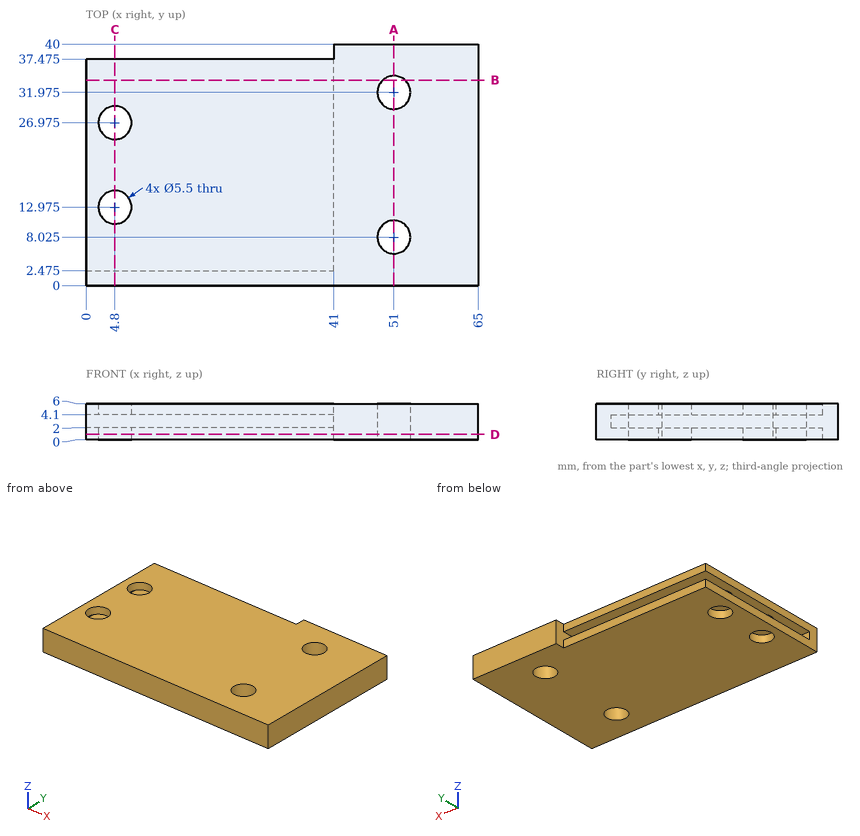
Source: three-view drawing plus pictorial views. Frame: mm from the lowest corner of the part. Give positions to 0.01 mm unless a question says otherwise; leave off trailing zeros. Write each loop counter-clockwise with the first axis right and the second up, starting at its lowest first coordinate (ties: lowest second). Pieces come first, ordered by that corner, then holes. Notation, with made-up numbers: M -4.75,82.25 L 44.25,82.25 A25 ccw 44.25,95.25 Z; hole C 32,49 d10. An arc over 180 degrees is marked long. Use one line per item in the form item = value.
1. Cut plane D-D on z = 0.9. Return loops of the section in (x, y) (3 decimals).
Outcome:
outline = M 0,0 L 65,0 L 65,40 L 41,40 L 41,37.475 L 0,37.475 Z; hole C 4.8,12.975 d5.5; hole C 4.8,26.975 d5.5; hole C 51,8.025 d5.5; hole C 51,31.975 d5.5
2. Cut plane A-A on x = 51. Return loops of the section in (y, z) (3 decimals), and give its area (3 significant figures).
Outcome:
outline = M 0,0 L 5.275,0 L 5.275,6 L 0,6 Z; M 10.775,0 L 29.225,0 L 29.225,6 L 10.775,6 Z; M 34.725,0 L 40,0 L 40,6 L 34.725,6 Z
area = 174 mm²
3. Cut plane C-C on x = 4.8. Return loops of the section in (y, z) (3 decimals), and give its area (3 significant figures).
Outcome:
outline = M 0,0 L 10.225,0 L 10.225,2 L 2.475,2 L 2.475,4.1 L 10.225,4.1 L 10.225,6 L 0,6 Z; M 15.725,0 L 24.225,0 L 24.225,2 L 15.725,2 Z; M 15.725,4.1 L 24.225,4.1 L 24.225,6 L 15.725,6 Z; M 29.725,0 L 37.475,0 L 37.475,2 L 29.725,2 Z; M 29.725,4.1 L 37.475,4.1 L 37.475,6 L 29.725,6 Z
area = 108 mm²
4. Cut plane B-B on y = 34. Return loops of the section in (x, z), and give its area (3 significant figures).
Outcome:
outline = M 0,0 L 49.14,0 L 49.14,6 L 0,6 L 0,4.1 L 41,4.1 L 41,2 L 0,2 Z; M 52.86,0 L 65,0 L 65,6 L 52.86,6 Z
area = 282 mm²
5. First-contact query: P1, Ø5, axis at x = 4.8, y = 12.975, coming from the +Z side; P2, Ø2.5, axis at x = 28.5, z = 3.5, coming from the +Y side (3 decimals). Flat tips, straight axial feed; report the tip coordinate or a pass-through.
Outcome:
P1 = through
P2 = 37.475
6. Ray query, L1, parallel to Y at x = 4.8, z = 5.55 (3 decimals); L2, parallel to Z at x = 20.5, y = 24.5; L3, parallel to X at y = 32, z = 0.7. Return the intervals inside material, ascending.
Outcome:
L1 = 0 to 10.225, 15.725 to 24.225, 29.725 to 37.475
L2 = 0 to 2, 4.1 to 6
L3 = 0 to 48.25, 53.75 to 65
